Check sheet for the modelled part. Datum: model origin and axes. Units: mm. Face numbers are marked on the shaded views. A direction names the side the tool comes from. Coordinates: 2 decimals unless noted, no trailing zeros. Loops run counter-clockwise (first coordinate to the right, second up) from the corner with the lowest first, then second, coordinate; pieces in that order, holes last. Notation, with made-up numbers: M -31.5,82.5 L -13.5,82.5 A24 ccw -13.5,93.5 Z; hole C 30.5,-3 d4. An arc over 180 degrees is marked long. Write each question's results on one line, items separated by ' | '. Start each with the question number.
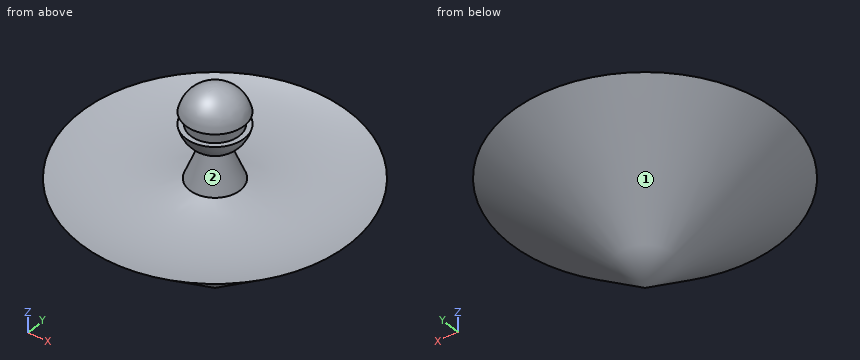
from build123d import *


with BuildPart() as f1:
    # F0 (on Front) → F1 (revolve)
    with BuildSketch(Plane.XZ):
        with BuildLine():
            Line((-41.350949, 15.48482), (-43.916382, 21.997772))
            ThreePointArc((-43.916382, 21.997772), (-41.694805, 23.730102), (-40.499528, 26.281119))
            Line((-40.499528, 26.281119), (-40.512723, 26.281119))
            Line((-40.512723, 26.281119), (-41.512723, 26.281119))
            Line((-41.512723, 26.281119), (-41.512723, 28.781119))
            Line((-41.512723, 28.781119), (-40.512723, 28.781119))
            ThreePointArc((-40.512723, 28.781119), (-42.625913, 32.205739), (-46.420603, 33.545113))
            Line((-46.420603, 33.545113), (-46.420603, -6.454887))
            Line((-46.420603, -6.454887), (-19.350949, 15.48482))
            ThreePointArc((-19.350949, 15.48482), (-30.350949, 13.892111), (-41.350949, 15.48482))
        make_face()
    revolve(axis=Axis((-46.420603, 0, 13.545113), (0, 0, -1)))


solid = f1.part
1) Thickness scan on probe 1 along Y at (x, z) = (-42.5, 27); probe 2 along Y at (x, z) = (-55, 12); probe 3 along Z at (x, y) = (-55, -18.5). Record the ranges inside material, lowest first.
2) Section check A-A (z = 23.5). Enter the section's corners in (x, y).
3) Set-up check for the marked faces 1 and 2: record each of +Z, -Z, +X, -X, +Y, -Y from which the full face is reachable in a straight line by a thin tool's end or side.
4) Gauge pin test, flat ends, axial feed: P1, Ø8, axis at x = -51, z = 12.5, coming from the +Y side; P2, Ø1, axis at x = -61.5, y = -14.5, coming from the -Z side; P3, Ø2, axis at x = -55, y = 3.5, coming from the -Z side. Record the tip position at first contact, or that the pin passes through.
Return value:
1) probe 1: y = -2.95 to 2.95 | probe 2: y = -21.09 to 21.09 | probe 3: z = 10.07 to 14.13
2) outline: C -46.42,0 d9.07
3) face 1: -Z | face 2: none
4) P1: stops at y = 27 | P2: stops at z = 10.1 | P3: stops at z = 0.24
